Design review of the part built by this model. Coordinates are the model's own, in mm. A direction names the side the tool comes from. Give positions to 0.01 mm unless a question says otherwise; leave off trailing zeros. Order: outer loops, then holes, each group sorted by start corner. A loop starts at its lowest first (then second) coordinate and runs counter-clockwise, first axis right, second up. Notation, with made-up numbers: M -19,35 L 5,35 A26 cw 5,71 Z; hole C 23.25,-28 d11. An arc over 180 degrees is marked long. Put each result on its own line as item: value. Start each with the question number.
from build123d import *

# Parameters (mm, degrees)
BOSS_EXTRUDE1_DEPTH = 190
CUT_EXTRUDE1_START  = 5
CUT_EXTRUDE1_DEPTH  = 182
FILLET3_START       = -1
FILLET3_DEPTH       = 192
CUT_EXTRUDE3_DEPTH  = 203
FILLET4_R           = 0.5
FILLET5_R           = 2
FILLET6_R           = 2


with BuildPart() as part:
    # Sketch1 → Boss-Extrude1 (new body)
    with BuildSketch(Plane.XY):
        Polygon((0, 0), (19, 0), (19, 5), (6.83805717, 10.67120708), (-6.91649822, 22.212649435), (-16, 29.600046382), (-16, 12.189630226), (-16, 5), (0, 5), align=None)
    extrude(amount=BOSS_EXTRUDE1_DEPTH)

    # Sketch2 → Cut-Extrude1 (cut)
    with BuildSketch(Plane.XY.offset(CUT_EXTRUDE1_START)):
        Polygon((21.633927393, 1.359461681), (3.507771652, 9.811826915), (2.873844259, 8.452365235), (21, 0), align=None)
    extrude(amount=CUT_EXTRUDE1_DEPTH, mode=Mode.SUBTRACT)

    # Fillet3: read off the stored shape, not the designer's step
    # Fillet3 outline → Fillet3 (cut)
    with BuildSketch(Plane.XY.offset(FILLET3_START)):
        with BuildLine():
            Line((19, 5), (9.753768459, 9.311588577))
            ThreePointArc((9.753768459, 9.311588577), (15.206282278, 5.479370881), (19, 0))
            Line((19, 0), (19, 5))
        make_face()
    extrude(amount=FILLET3_DEPTH, mode=Mode.SUBTRACT)

    # Sketch6 → Cut-Extrude3 (cut)
    with BuildSketch(Plane.XY.offset(190)):
        Polygon((0, 1.071241245), (15.85883014, 0), (18.190743079, 1.570510584), (20.776431757, 1.395851019), (18.077940116, -2.328162287), (-1.219539475, -1.555674607), (-2.427097473, 0.237321984), align=None)
    extrude(amount=-CUT_EXTRUDE3_DEPTH, mode=Mode.SUBTRACT)

    # Fillet4
    fillet4_edges = [part.edges().sort_by_distance(p)[0] for p in [
        (16.849447034, 3.590501512, 96),
    ]]
    fillet(fillet4_edges, radius=FILLET4_R)

    # Fillet5
    fillet5_edges = [part.edges().sort_by_distance(p)[0] for p in [
        (15.85883014, 0, 95),
    ]]
    fillet(fillet5_edges, radius=FILLET5_R)

    # Fillet6
    fillet6_edges = [part.edges().sort_by_distance(p)[0] for p in [
        (-16, 29.600046382, 95),
    ]]
    fillet(fillet6_edges, radius=FILLET6_R)


solid = part.part
1. Consider section B-B on x = -9. Give the boundary of the cut face in (y, z), then the cut area to 3 significant figures.
2. Consider section C-C on y = 16. Give the boundary of the cut face in (x, z).
3. The part is to be moulded in two halves that separate along Z. For faces 4 (the flat face through (10, 6, 187)), 5 (the cylindrical face through (-14.831, 27.215, 96.33)), 6 (the flat face through (-3, 11, 0)), say which applies: +Z half, -Z half, draft (parallel to the pull), parting line (faces both ways), or undercut.
4. Insertion check: pin 1 (1.5 mm diameter, centred on y = 9, z = 146, fed in from +X); pin 2 (2 mm diameter, centred on x = 0, z = 166, fed in from +Y); pin 3 (5 mm diameter, centred on x = -12.5, z = 56, fed in from -Y). Each pin has a flat end and moves straight along its axis. Give the tip position at first contact, or say it passes through.
5. Consider section A-A on z = 113. Give the boundary of the cut face in (x, y).
6. To check wall thickness, follow probe 1 along X at (y, z) = (15.5, 103); probe 2 along Y at (x, z) = (13, 30); probe 3 along Y at (x, z) = (6, 73). State the ranges of each line that lie inside material, in increasing order.
7. Machinability: for faces 1 (the flat face through (10.312, 4.984, 94.726)), 2 (the flat face through (-16, 15, 94)), 3 (the flat face through (0, 3, 94)), which of the approach directions +Z, -Z, +X, -X, +Y, -Y give a long, thin tool a straight path to every point of the face, cutting with its end or side? Answer none if there is none.
Returned:
1. outline: M 5,0 L 23.91,0 L 23.91,190 L 5,190 Z
1. area: 3,590 mm2
2. outline: M -16,0 L 0.49,0 L 0.49,190 L -16,190 Z
3. face 4: undercut
3. face 5: draft
3. face 6: -Z half
4. pin 1: stops at x = 11.72
4. pin 2: stops at y = 17.25
4. pin 3: stops at y = 5
5. outline: M -16,5 L 0,5 L 0,1.07 L 15.18,0.05 A2 ccw 16.43,0.38 L 17.96,1.42 L 2.87,8.45 L 3.51,9.81 L 14.74,4.58 A0.5 ccw 15.31,5.38 A19 ccw 9.75,9.31 L 6.84,10.67 L -6.92,22.21 L -12.74,26.95 A2 ccw -16,25.4 Z
6. probe 1: x = -16 to 1.08
6. probe 2: y = 0.19 to 3.73, 5.39 to 7.38
6. probe 3: y = 0.67 to 6.99, 8.65 to 11.37
7. face 1: none
7. face 2: +Z, -Z, -X, +Y, -Y
7. face 3: +Z, -Z, -X, -Y
